Source: three-view drawing plus pictorial views. Frame: mm from the lowest corner of the part. Coordinates: 2 decimals unless noted, no trailing zeros. Order: outer loops, then holes, each group sorted by start corner. A loop starts at its lowest first (then second) coordinate and runs counter-clockwise, first axis right, second up. Notation, with made-up numbers: (-37.75, -2.5) - (13.25, -2.5) arc R27 cw to (13.25, 25.5) - close; hole circle Ø6 at (34.5, -18.75). An arc over 180 degrees is marked (long way). One line per question, with ' | ' between items.
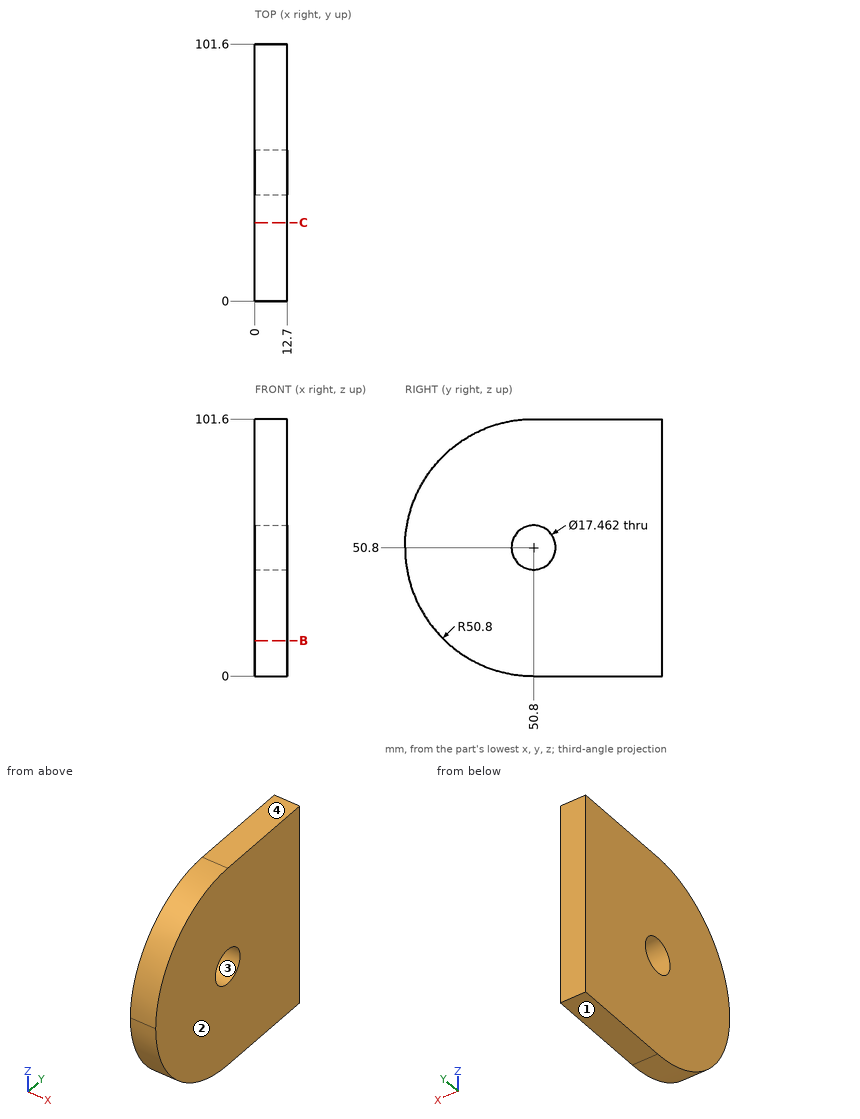
Item 1: Ray query, line 1 (Z direction, x = 7.25, y = 50.8); line 2 (Y direction, x = 4.75, z = 48.5). Return the intervals inside material, ascending.
Data:
line 1: 0 to 42.07, 59.53 to 101.6 | line 2: 0.05 to 42.38, 59.22 to 101.6
Item 2: Section B-B on z = 14. Return the cut outline in (x, y).
Data:
outline: (0, 15.78) - (12.7, 15.78) - (12.7, 101.6) - (0, 101.6) - close
Item 3: Contact query for a flat-ended pin moving along its axis: P1, Ø4, axis at x = 8, y = 20.5, coming from the +Z side. Output: stop coordinate, or through.
Data:
P1: z = 92.99
Item 4: Draft query along Z for the marked faces 1, 2, 3 and 4. Return one class per face: released by +Z, released by -Z, zero draft, split by the parting line, or undercut.
Data:
face 1: released by -Z | face 2: zero draft | face 3: undercut | face 4: released by +Z
Item 5: Section C-C on y = 31. Return the cut outline in (x, z), and give its area (3 significant figures).
Data:
outline: (0, 4.02) - (12.7, 4.02) - (12.7, 97.58) - (0, 97.58) - close | area: 1,190 mm^2
